from build123d import *

# Parameters (mm, degrees)
F0_W     = 1
F0_H     = 1
F0_W_2   = 3.75
F0_H_2   = 7.8
F0_R     = 0.5
F1_DEPTH = 2.5
F2_W     = 3.75
F2_H     = 7.8
F2_R     = 0.5
F3_DEPTH = 11.5
F4_W     = 1
F4_H     = 1
F5_DEPTH = 2


with BuildPart() as f1:
    # F0 (on Top) → F1 (new body)
    with BuildSketch(Plane.XY):
        Polygon((-15.375, 3.9), (-11.625, 3.9), (-11.625, -3.9), (-0.625, 0), (0.375, 0), (11.625, -3.9), (11.625, 3.9), (15.375, 3.9), (0.375, 7.65), (0.375, 6.65), (-0.625, 6.65), (-0.625, 7.65), align=None)
        with Locations((-0.125, 7.15)):
            Rectangle(F0_W, F0_H)
        with Locations((-13.5, 0)):
            Rectangle(F0_W_2, F0_H_2)
        with Locations((-13.5, 0)):
            Circle(F0_R, mode=Mode.SUBTRACT)
        with Locations((13.5, 0)):
            Rectangle(F0_W_2, F0_H_2)
        with Locations((13.5, 0)):
            Circle(F0_R, mode=Mode.SUBTRACT)
    extrude(amount=F1_DEPTH)

    # F2 (on face) → F3 (join)
    with BuildSketch(Plane.XY.offset(2.5)):
        with Locations((-13.5, 0)):
            Rectangle(F2_W, F2_H)
        with Locations((-13.5, 0)):
            Circle(F2_R, mode=Mode.SUBTRACT)
        with Locations((13.5, 0)):
            Rectangle(F2_W, F2_H)
        with Locations((13.5, 0)):
            Circle(F2_R, mode=Mode.SUBTRACT)
    extrude(amount=F3_DEPTH)

    # F4 (on face) → F5 (join)
    with BuildSketch(Plane.XY.offset(2.5)):
        with Locations((-0.125, 7.15)):
            Rectangle(F4_W, F4_H)
    extrude(amount=F5_DEPTH)


solid = f1.part
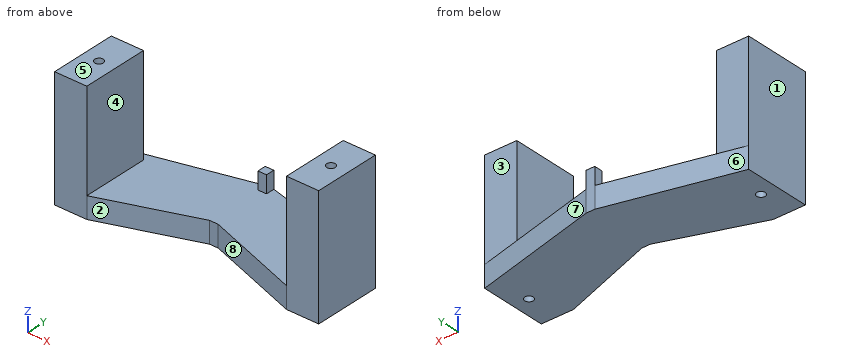
The listing builds one solid part. Answer for the finished solid, in the listing's coordinates (mm). Face numbers are marked on the shaded views. A direction names the side the tool comes from. Round coordinates to 2 decimals unless told otherwise and drop trailing zeros. Write each loop counter-clockwise with the first axis right and the second up, starting at its lowest first coordinate (ties: lowest second). Pieces come first, ordered by that corner, then holes. Notation, with made-up numbers: M 29,67 L 75,67 A35 ccw 75,106 Z; hole C -12.75,-22 d7. An arc over 180 degrees is marked long. Write each question's results on one line, items separated by ' | '. Start each with the question number.
(1) Find the intervals of material crossed by line 1 (X direction, y = 1.75, z = 9) (3 decimals); line 2 (Z direction, x = 10, y = -1.75); line 3 (Y direction, x = -12.5, z = 1.75), in increasing order.
(2) The part is cut by section B-B, the plane z = 6.25. Write down the section's boundary in (x, y) (3 decimals), and give its area (3 significant figures).
(3) The part is cut by section D-D, the plane x = -13.5. Write down the section's boundary in (y, z).
(4) The part is cut by section C-C, the plane y = 2.5. Write down the section's boundary in (x, z) (3 decimals), and give its area (3 significant figures).
(5) Each of these flat-tipped pins is pushed along its axis until it touches: P1, Ø0.5, axis at y = 7, z = 4, coming from the +X side (3 decimals); P2, Ø3, axis at x = -13, z = 9, coming from the +Y side; P3, Ø1.5, axis at x = 6.5, y = 0.5, coming from the +Z side. Where does it stop, or does it pass through?
(6) The part is cut by section A-A, the plane z = 4. Write down the section's boundary in (x, y) (3 decimals), and give its area (3 significant figures).
(7) For the marked faces 1, 2, 3, 4 and 5, determine the directions among +Z, -Z, +X, -X, +Y, -Y from which every point of the face is accessible in a straight line to the end or side of a thin tool.
(8) Determine the mould class of the marked faces 6, 7 and 8 for opening direction X: +X half, -X half, draft (parallel to the pull), parting line (faces both ways), or undercut.
Worked answers:
1) line 1: x = -15.375 to -11.625, 11.625 to 15.375 | line 2: z = 0 to 2.5 | line 3: y = -3.9 to 4.63
2) outline: M -15.375,-3.9 L -11.625,-3.9 L -11.625,3.9 L -15.375,3.9 Z; M 11.625,-3.9 L 15.375,-3.9 L 15.375,3.9 L 11.625,3.9 Z; hole C -13.5,0 d1; hole C 13.5,0 d1 | area: 56.9 mm²
3) outline: M -3.9,0 L -0.5,0 L -0.5,14 L -3.9,14 Z; M 0.5,0 L 4.38,0 L 4.38,2.5 L 3.9,2.5 L 3.9,14 L 0.5,14 Z
4) outline: M -15.375,0 L 15.375,0 L 15.375,14 L 11.625,14 L 11.625,2.5 L -11.625,2.5 L -11.625,14 L -15.375,14 Z | area: 163 mm²
5) P1: stops at x = 0.375 | P2: stops at y = 3.9 | P3: stops at z = 2.5
6) outline: M -15.375,-3.9 L -11.625,-3.9 L -11.625,3.9 L -15.375,3.9 Z; M -0.625,6.65 L 0.375,6.65 L 0.375,7.65 L -0.625,7.65 Z; M 11.625,-3.9 L 15.375,-3.9 L 15.375,3.9 L 11.625,3.9 Z; hole C -13.5,0 d1; hole C 13.5,0 d1 | area: 57.9 mm²
7) face 1: +Z, -Z, -X, +Y, -Y | face 2: +Z, -Z, -Y | face 3: +Z, +X, -X, +Y | face 4: +Z, +Y, -Y | face 5: +Z, +X, -X, +Y, -Y
8) face 6: -X half | face 7: +X half | face 8: undercut
